```python
from build123d import *

# Parameters (mm, degrees)
SKETCH_1_W      = 10
SKETCH_1_H      = 15
SKETCH_1_R      = 2
EXTRUDE_1_DEPTH = 2.5
FILLET_1_R      = 1


with BuildPart() as part:
    # ｽｹｯﾁ1 → ﾎﾞｽ - 押し出し1 (new body)
    with BuildSketch(Plane.XY):
        Rectangle(SKETCH_1_W, SKETCH_1_H)
        Circle(SKETCH_1_R, mode=Mode.SUBTRACT)
    extrude(amount=EXTRUDE_1_DEPTH)

    # ﾌｨﾚｯﾄ1
    fillet_1_edges = [part.edges().sort_by_distance(p)[0] for p in [
        (5, -7.5, 1.25),
        (-5, -7.5, 1.25),
        (-5, 7.5, 1.25),
        (5, 7.5, 1.25),
    ]]
    fillet(fillet_1_edges, radius=FILLET_1_R)


solid = part.part
```
Work out the finished part from the listing and answer in its coordinate system (mm). Round coordinates to 2 decimals unless told otherwise and drop trailing zeros. Write each loop counter-clockwise with the first axis right and the second up, starting at its lowest first coordinate (ties: lowest second). Pieces come first, ordered by that corner, then holes.
1) Determine the mould class of faces 1 (the face through (-4.715, 7.199, 1.268)), 2 (the face through (0, -2, 1)), 3 (the face through (5, 0, 1)) for opening direction X: pulls with the +X half, pulls with the -X half, needs draft (parallel to the pull), parting line crosses it, or undercut.
2) A cutting plane is placed at C-C on x = 0. Determine the outline of the cut face in (y, z), and give its area (3 significant figures).
3) A flat-ended cylindrical pin translates along its axis: P1, Ø3, axis at x = 0, y = 0, coming from the -Z side. Find the tip coordinate at first contact, or state that the pin passes through.
4) Consider probe 1 along Y at (x, z) = (0, 1.8); probe 2 along Y at (x, z) = (-1, 1.55); probe 3 along X at (y, z) = (1, 0.7). Determine where each line is inside the solid, lowest interval first.
5) A cutting plane is placed at A-A on y = 0. Determine the outline of the cut face in (x, z).
6) A cutting plane is placed at B-B on z = 0.35. Determine the outline of the cut face in (x, y), and give its area (3 significant figures).
Entries:
1. face 1: pulls with the -X half
1. face 2: undercut
1. face 3: pulls with the +X half
2. outline: (-7.5, 0) - (-2, 0) - (-2, 2.5) - (-7.5, 2.5) - close; (2, 0) - (7.5, 0) - (7.5, 2.5) - (2, 2.5) - close
2. area: 27.5 mm2
3. P1: passes through
4. probe 1: y = -7.5 to -2, 2 to 7.5
4. probe 2: y = -7.5 to -1.73, 1.73 to 7.5
4. probe 3: x = -5 to -1.73, 1.73 to 5
5. outline: (-5, 0) - (-2, 0) - (-2, 2.5) - (-5, 2.5) - close; (2, 0) - (5, 0) - (5, 2.5) - (2, 2.5) - close
6. outline: (-5, -6.5) arc R1 ccw to (-4, -7.5) - (4, -7.5) arc R1 ccw to (5, -6.5) - (5, 6.5) arc R1 ccw to (4, 7.5) - (-4, 7.5) arc R1 ccw to (-5, 6.5) - close; hole circle Ø4 at (0, 0)
6. area: 137 mm2
